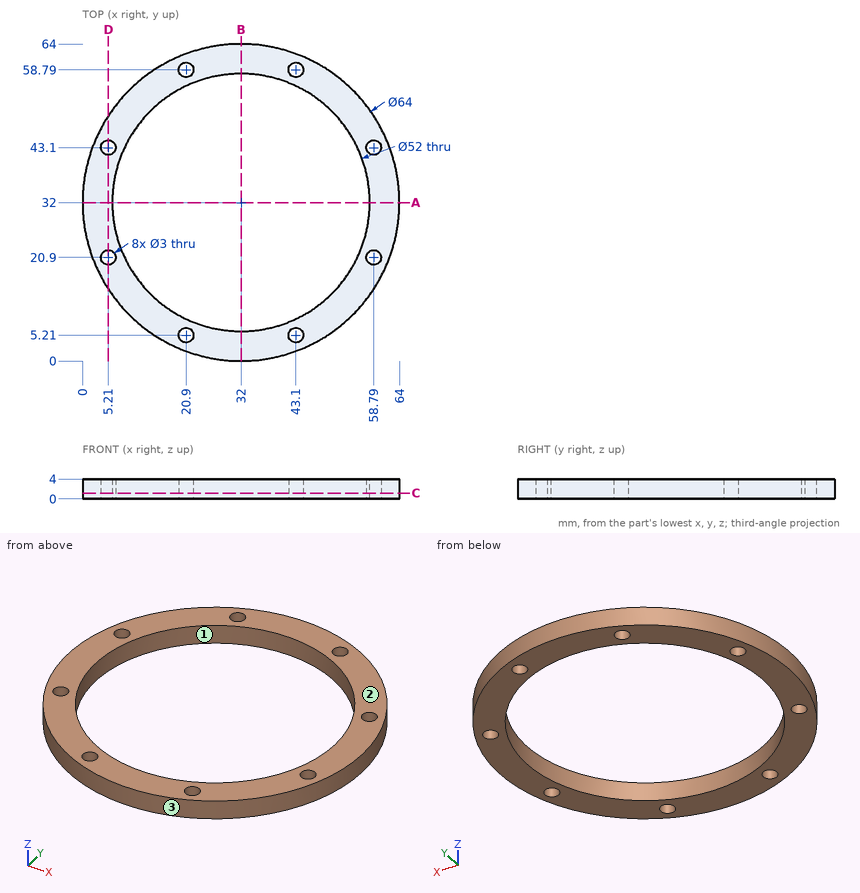
Here's the drawing with two shaded views (mm, measured from the low corner). I have some questions. Round coordinates to 2 decimals unless told otherwise and drop trailing zeros. Write each loop counter-clockwise with the first axis right and the second up, starting at its lowest first coordinate (ties: lowest second). Pieces come first, ordered by that corner, then holes.
(1) Thinking about a two-plate mould opening in X: for the marked faces 1, 2 and 3, which applies, +X half, -X half, draft (parallel to the pull), parting line (faces both ways), or undercut?
Findings below:
face 1: undercut
face 2: draft
face 3: parting line
(2) Suppose I cut it at A-A on y = 32. Write out the boundary of the cut face in (x, z).
Findings below:
outline: (0, 0) - (6, 0) - (6, 4) - (0, 4) - close; (58, 0) - (64, 0) - (64, 4) - (58, 4) - close
(3) Suppose I cut it at C-C on z = 1.15. State how many separate pieces and enclosed holes the cut face has, and give its area (3 significant figures).
Findings below:
separate pieces: 1
enclosed holes: 9
area: 1,040 mm2
(4) If I drill on probe 1 along Y at (x, z) = (32, 2.55); probe 2 along X at (y, z) = (43.5, 3.65); probe 3 along X at (y, z) = (43.1, 2.6), over which ranges is the centre line in solid material (lowest first)?
Findings below:
probe 1: y = 0 to 6, 58 to 64
probe 2: x = 2.14 to 3.76, 6.66 to 8.68, 55.32 to 57.34, 60.24 to 61.86
probe 3: x = 1.99 to 3.71, 6.71 to 8.49, 55.51 to 57.29, 60.29 to 62.01
(5) Suppose I cut it at D-D on x = 5.21. Write out the boundary of the cut face in (y, z).
Findings below:
outline: (14.5, 0) - (19.4, 0) - (19.4, 4) - (14.5, 4) - close; (22.4, 0) - (41.6, 0) - (41.6, 4) - (22.4, 4) - close; (44.6, 0) - (49.5, 0) - (49.5, 4) - (44.6, 4) - close
